from build123d import *

# Parameters (mm, degrees)
CROQUIS1_R              = 2.5
SALIENTE_EXTRUIR1_DEPTH = 3


with BuildPart() as part:
    # Croquis1 → Saliente-Extruir1 (new body)
    with BuildSketch(Plane.XY):
        with BuildLine():
            Line((-12.5, -30), (-7.5, -30))
            Line((-7.5, -30), (-7.5, -27))
            Line((-7.5, -27), (-2.5, -27))
            Line((-2.5, -27), (-2.5, -30))
            Line((-2.5, -30), (2.5, -30))
            Line((2.5, -30), (2.5, -27))
            Line((2.5, -27), (7.5, -27))
            Line((7.5, -27), (7.5, -30))
            Line((7.5, -30), (12.5, -30))
            Line((12.5, -30), (12.5, -27))
            Line((12.5, -27), (17.5, -27))
            Line((17.5, -27), (17.5, 30))
            ThreePointArc((17.5, 30), (0, 47.5), (-17.5, 30))
            Line((-17.5, 30), (-17.5, -27))
            Line((-17.5, -27), (-12.5, -27))
            Line((-12.5, -27), (-12.5, -30))
        make_face()
        with Locations((0, 30)):
            Circle(CROQUIS1_R, mode=Mode.SUBTRACT)
    extrude(amount=SALIENTE_EXTRUIR1_DEPTH)


solid = part.part
Design review of the part built by this model. Coordinates are the model's own, in mm. A direction names the side the tool comes from. Coordinates: 2 decimals unless noted, no trailing zeros. Loops run counter-clockwise (first coordinate to the right, second up) from the corner with the lowest first, then second, coordinate; pieces in that order, holes last. Notation, with made-up numbers: M -18,26 L 36,26 A16 cw 36,34 Z; hole C 47.25,34 d4. An arc over 180 degrees is marked long. Use one line per item in the form item = value.
(1) Draft analysis for pull direction X (two halves, no side actions). For faces 4 (the face through (2.5, -29, 1)), 5 (the face through (-17.5, 2, 1)), 6 (the face through (5, -27, 1)), 7 (the face through (10, -30, 1)), state which applies: pulls with the +X half, pulls with the -X half, needs draft (parallel to the pull), parting line crosses it, or undercut.
Return value:
face_4 = undercut
face_5 = pulls with the -X half
face_6 = undercut
face_7 = needs draft
(2) For line 1 along Y through (x, z) = (0, 1.2); line 2 along Y through (x, z) = (-2, 0.9); line 3 along X through (y, z) = (28, 1.85), list the stretches that pass through material, from the lowest coordinate up. Write a range as from..to.
Return value:
line_1 = -30..27.5, 32.5..47.5
line_2 = -30..28.5, 31.5..47.39
line_3 = -17.5..-1.5, 1.5..17.5
(3) Consider section C-C (y = 36.5). Write out the cut boundary in (x, z).
Return value:
outline = M -16.25,0 L 16.25,0 L 16.25,3 L -16.25,3 Z
(4) Consider section A-A (z = 2.5). Write out the cut boundary in (x, y).
Return value:
outline = M -17.5,-27 L -12.5,-27 L -12.5,-30 L -7.5,-30 L -7.5,-27 L -2.5,-27 L -2.5,-30 L 2.5,-30 L 2.5,-27 L 7.5,-27 L 7.5,-30 L 12.5,-30 L 12.5,-27 L 17.5,-27 L 17.5,30 A17.5 ccw -17.5,30 Z; hole C 0,30 d5
(5) For faces 1 (the face through (12.5, -29, 1)), 2 (the face through (-15, -27, 1)), 3 (the face through (-5, -27, 1)), list the 3-axis set-ups (+Z, -Z, +X, -X, +Y, -Y) from which the entire face can be reached by the end or side of a thin tool; tool diameter is ignored.
Return value:
face_1 = +Z, -Z, +X, -Y
face_2 = +Z, -Z, -X, -Y
face_3 = +Z, -Z, -Y
(6) Clearance check with flat-ended pins moving along their axes: P1, Ø1.5, axis at y = -28.5, z = 1, coming from the -X side; P2, Ø1, axis at x = -1.5, y = -6, coming from the -Z side; P3, Ø0.9, axis at y = -28.5, z = 1.5, coming from the +X side; P4, Ø1.5, axis at x = -5, z = 1, coming from the -Y side. State where each tip first meets the part, or that it passes through.
Return value:
P1 = -12.5
P2 = 0
P3 = 12.5
P4 = -27
(7) Consider section D-D (x = -14). Write out the cut boundary in (y, z), and give its area (4 significant figures).
Return value:
outline = M -27,0 L 40.5,0 L 40.5,3 L -27,3 Z
area = 202.5 mm2
(8) Consider section B-B (x = 0). Write out the cut boundary in (y, z), and give its area (4 significant figures).
Return value:
outline = M -30,0 L 27.5,0 L 27.5,3 L -30,3 Z; M 32.5,0 L 47.5,0 L 47.5,3 L 32.5,3 Z
area = 217.5 mm2
